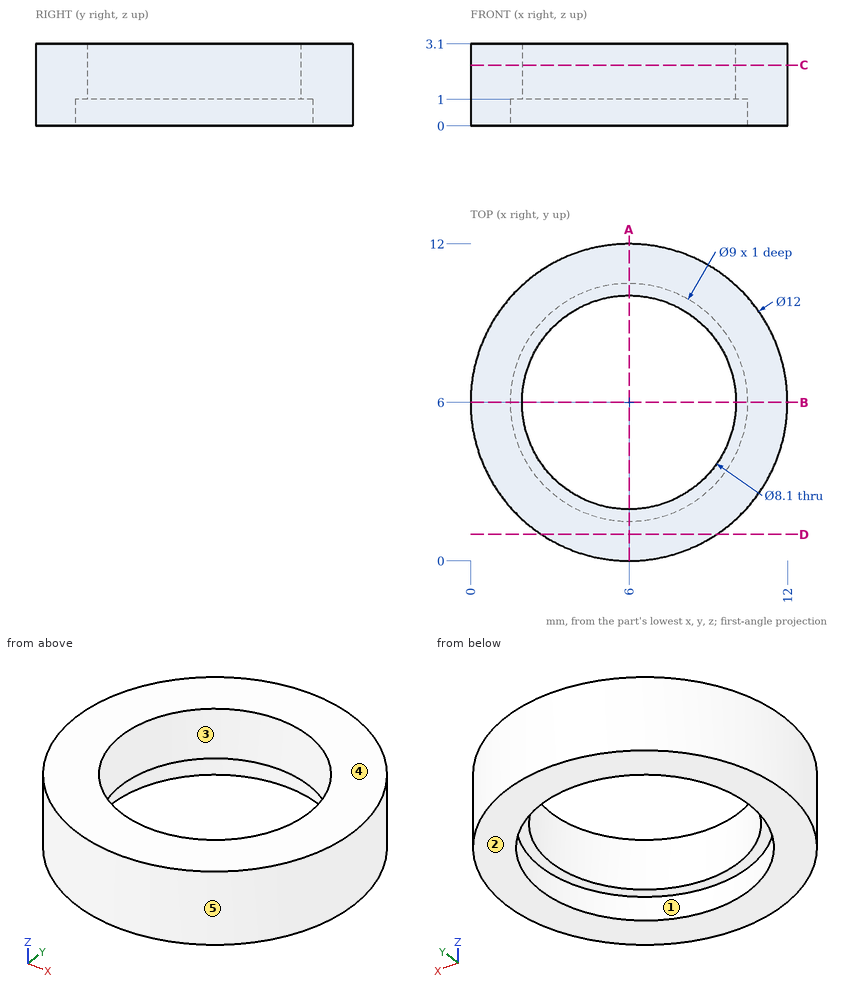
Verification items for this drawing (mm, ordinates from the low corner). A direction names the side the tool comes from. Give positions to 0.01 mm unless a question says otherwise; leave off trailing zeros. Write each loop counter-clockwise with the first axis right and the second up, starting at its lowest first coordinate (ties: lowest second). Pieces come first, ordered by that corner, then holes. Notation, with made-up numbers: (15, 39.5) - (40, 39.5) arc R25 cw to (40, 53.5) - close; hole circle Ø2 at (15.25, 16.5). An arc over 180 degrees is marked (long way). Answer as CSV lines item,"result". Start each with the question number.
1. Thickness scan on line 1 (Y direction, x = 6, z = 0.85); line 2 (Y direction, x = 6, z = 2.55); line 3 (X direction, y = 2.75, z = 2.05). Record the ranges inside material, lowest first.
2. Sectioned sample at A-A (x = 6). Record the boundary of the cut face in (y, z).
3. Sectioned sample at C-C (z = 2.3). Record the boundary of the cut face in (x, y).
4. Sectioned sample at D-D (y = 1). Record the boundary of the cut face in (x, z), then the cut area to 3 significant figures.
5. Set-up check for the marked faces 1 and 2: record each of +Z, -Z, +X, -X, +Y, -Y from which the full face is reachable in a straight line by a thin tool's end or side.
6. Draft check along Y on the marked faces 3, 4 and 5. Enter one of: pulls with the +Y half, pulls with the -Y half, needs draft (parallel to the pull), parting line crosses it, or undercut.
Derived:
1,line 1,"0 to 1.5, 10.5 to 12"
1,line 2,"0 to 1.95, 10.05 to 12"
1,line 3,"0.96 to 3.58, 8.42 to 11.04"
2,outline,"(0, 0) - (1.5, 0) - (1.5, 1) - (1.95, 1) - (1.95, 3.1) - (0, 3.1) - close; (10.05, 1) - (10.5, 1) - (10.5, 0) - (12, 0) - (12, 3.1) - (10.05, 3.1) - close"
3,outline,"circle Ø12 at (6, 6); hole circle Ø8.1 at (6, 6)"
4,outline,"(2.68, 0) - (9.32, 0) - (9.32, 3.1) - (2.68, 3.1) - close"
4,area,"20.6 mm²"
5,face 1,"-Z"
5,face 2,"-Z, +X, -X, +Y, -Y"
6,face 3,"undercut"
6,face 4,"needs draft"
6,face 5,"parting line crosses it"
